```python
from build123d import *

# Parameters (mm, degrees)
CROQUIS1_R              = 2.5
SALIENTE_EXTRUIR1_DEPTH = 2.5
CROQUIS3_R              = 2.5
CROQUIS3_R_2            = 2
SALIENTE_EXTRUIR7_DEPTH = 5


with BuildPart() as part:
    # Croquis1 → Saliente-Extruir1 (new, symmetric)
    with BuildSketch(Plane.XY):
        with BuildLine():
            Line((-45, 6), (45, 6))
            ThreePointArc((45, 6), (51, 0), (45, -6))
            Line((45, -6), (-45, -6))
            ThreePointArc((-45, -6), (-51, 0), (-45, 6))
        make_face()
        with Locations((45, 0)):
            Circle(CROQUIS1_R, mode=Mode.SUBTRACT)
        with Locations((-45, 0)):
            Circle(CROQUIS1_R, mode=Mode.SUBTRACT)
    extrude(amount=SALIENTE_EXTRUIR1_DEPTH, both=True)

    # Croquis3 → Saliente-Extruir7 (add, through all)
    # profile 1 of 2: a face of its own
    with BuildSketch(Plane.XY.offset(2.5)):
        with Locations((-45, 0)):
            Circle(CROQUIS3_R)
        with Locations((-45, 0)):
            Circle(CROQUIS3_R_2, mode=Mode.SUBTRACT)
    # profile 2 of 2: a face of its own
    with BuildSketch(Plane.XY.offset(2.5)):
        with BuildLine():
            Line((-43.934051012, 1.692262614), (-43.934051012, 0))
            Line((-43.934051012, 0), (-43.934051012, -1.692262614))
            ThreePointArc((-43.934051012, -1.692262614), (-43.249014852, -0.966463146), (-43, 0))
            ThreePointArc((-43, 0), (-43.249014852, 0.966463146), (-43.934051012, 1.692262614))
        make_face()
    extrude(amount=-SALIENTE_EXTRUIR7_DEPTH)


solid = part.part
```
Can you work these out from the model? Positions are in its coordinate system, mm. A direction names the side the tool comes from. Give positions to 0.01 mm unless a question says otherwise; leave off trailing zeros. Loops run counter-clockwise (first coordinate to the right, second up) from the corner with the lowest first, then second, coordinate; pieces in that order, holes last. Notation, with made-up numbers: M 7.5,43 L 55.5,43 A13 cw 55.5,65 Z; hole C -12.75,-19 d1. An arc over 180 degrees is marked long. One line per question, with ' | ' between items. Start each with the question number.
Q1. If I drill on line 1 (Y direction, x = -45, z = -0.6); line 2 (Y direction, x = 45, z = -1.4); line 3 (X direction, y = -1, z = -2.3), over which ranges is the centre line in solid material (lowest first)? Write a range as from..to.
Q2. If we section it at C-C (y = 4.25): Please give me the cut outline in (x, z).
Q3. For faces 1 (the flat face through (-43.934, 0, 0)), 2 (the flat face through (-1, 0, -2.5)), which set-ups out of +Z, -Z, +X, -X, +Y, -Y let a thin tool reach every point of the face, with its end or its side?
Q4. If we section it at A-A (z = -1.05): Please give me the cut outline in (x, y), plus the area to 3 significant figures.
Q5. If we mould it in two halves opening along X, with no side actions, what happens to faces 3 (the cylindrical face through (-47, 0, 0)), 4 (the flat face through (1, -6, 0)), 5 (the cylindrical face through (51, 0, 0))? For each: +X half, -X half, draft (parallel to the pull), parting line (faces both ways), or undercut.
Q6. For pin 1 Ø4.5 at (x, y) = (45, 0) entering from +Z; pin 2 Ø2.5 at (x, y) = (-45, 0) entering from -Z; pin 3 Ø1.5 at (y, z) = (4.5, 1.5) entering from +X; pin 4 Ø1 at (y, z) = (-4, 0) entering from +X, each with a flat end and sliding along its axis, tell me the tip position at first contact or that it passes through.
Q7. If we section it at B-B (y = 0): Please give me the cut outline in (x, z), plus the area to 3 significant figures.
Computed:
1) line 1: y = -6..-2, 2..6 | line 2: y = -6..-2.5, 2.5..6 | line 3: x = -50.92..-46.73, -43.93..42.71, 47.29..50.92
2) outline: M -49.24,-2.5 L 49.24,-2.5 L 49.24,2.5 L -49.24,2.5 Z
3) face 1: +Z, -Z | face 2: -Z, +X, -X, +Y, -Y
4) outline: M -45,-6 L 45,-6 A6 ccw 45,6 L -45,6 A6 ccw Z; hole M -43.93,-1.69 L -43.93,1.69 A2 ccw long Z; hole C 45,0 d5 | area: 1,160 mm²
5) face 3: undercut | face 4: draft | face 5: +X half
6) pin 1: passes through | pin 2: stops at z = -2.5 | pin 3: stops at x = 49.68 | pin 4: stops at x = 49.87
7) outline: M -51,-2.5 L -47,-2.5 L -47,2.5 L -51,2.5 Z; M -43.93,-2.5 L 42.5,-2.5 L 42.5,2.5 L -43.93,2.5 Z; M 47.5,-2.5 L 51,-2.5 L 51,2.5 L 47.5,2.5 Z | area: 470 mm²
